Check sheet for the drawn part. Datum: minimum x, y, z corner. Units: mm. A direction names the side the tool comes from. Give positions to 0.01 mm unless a question says otherwise; leave off trailing zeros. Order: outer loops, then holes, each group sorted by start corner. A loop starts at its lowest first (then second) coordinate and runs counter-clockwise, first axis right, second up. Notation, with made-up numbers: (-7.75, -3.75) - (4.25, -3.75) arc R20 ccw to (4.25, 4.25) - close; hole circle Ø5 at (69.5, 69). An arc over 180 degrees is marked (long way). Answer as a JSON object with one key per item and string values. Group by question number.
(1) Thickness scan on line 1 (Y direction, x = 39, z = 83); line 2 (X direction, y = 2, z = 25); line 3 (X direction, y = 1, z = 66). Record the ranges inside material, lowest first.
(2) Mould release check, pull along Z, two halves, no side actions. Record for the marked faces 1, 2 and 3: +Z half, -Z half, draft (parallel to the pull), parting line (faces both ways), or undercut.
(3) Section check D-D (z = 56). Record the boundary of the cut face in (x, y).
(4) Depth check by flat-ended pin: pin 1 Ø3 at (y, z) = (21, 52) entering from -X; pin 2 Ø5 at (y, z) = (43, 66.5) entering from +X; pin 3 Ø8 at (x, y) = (78, 46) entering from -Z. Enter the tip coordinate at first touch or a pass-through.
(5) Access from +Z, -Z, +X, -X, +Y, -Y to the whole of each face (thin tool, end or side, straight path). Record for the marked faces 4 and 5.
(6) Section check C-C (x = 57). Record the boundary of the cut face in (y, z).
(7) Section check A-A (x = 25.5). Count the separate pieces of the cut face and the enclosed holes in it.
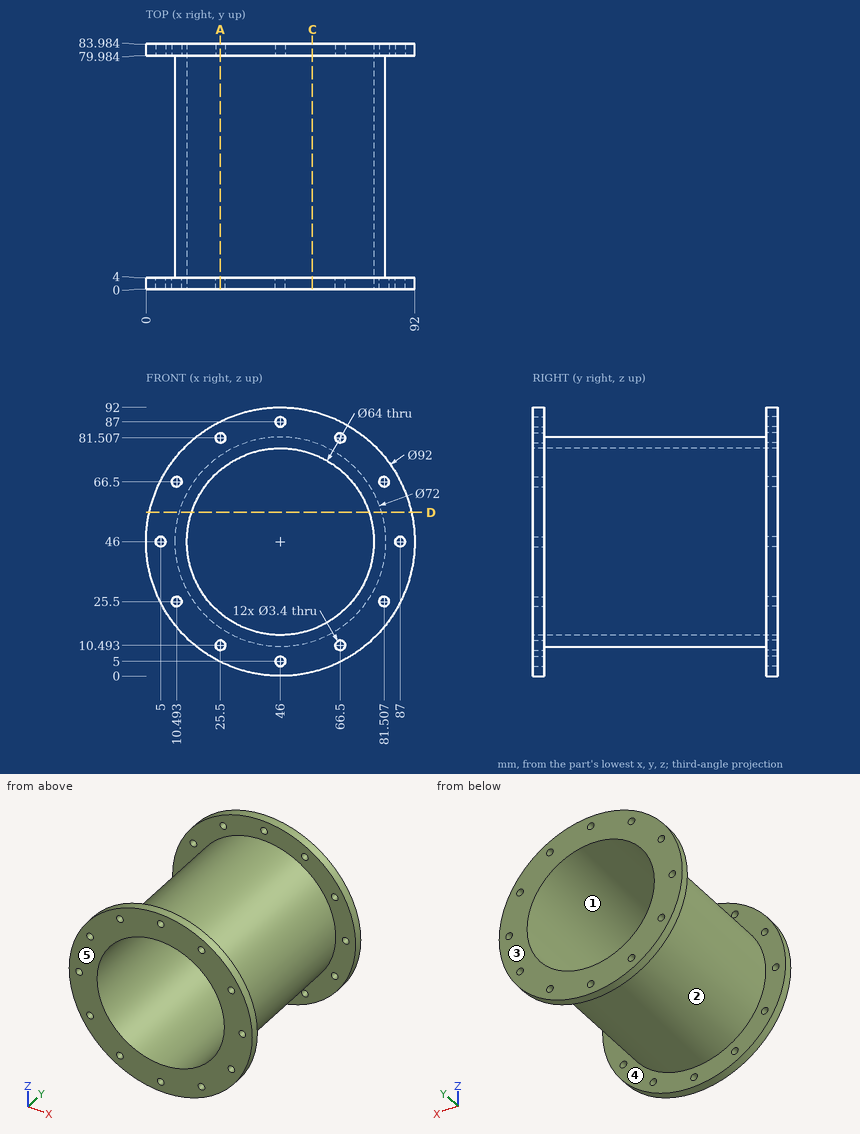
Solutions:
{
 "1": {"line 1": "y = 0 to 4, 79.98 to 83.98", "line 2": "x = 5.07 to 8.87, 12.12 to 21.85, 70.15 to 79.88, 83.13 to 86.93", "line 3": "x = 4.58 to 8.87, 12.12 to 21.02, 70.98 to 79.88, 83.13 to 87.42"},
 "2": {"face 1": "undercut", "face 2": "parting line", "face 3": "draft"},
 "3": {"outline": "(1.1, 0) - (15.6, 0) - (15.6, 83.98) - (1.1, 83.98) - (1.1, 79.98) - (11.42, 79.98) - (11.42, 4) - (1.1, 4) - close; (76.4, 0) - (90.9, 0) - (90.9, 4) - (80.58, 4) - (80.58, 79.98) - (90.9, 79.98) - (90.9, 83.98) - (76.4, 83.98) - close"},
 "4": {"pin 1": "stops at x = 10.28", "pin 2": "stops at x = 77.18", "pin 3": "stops at z = 23.37"},
 "5": {"face 4": "none", "face 5": "+Z, -Z, +X, -X, -Y"},
 "6": {"outline": "(0, 1.33) - (4, 1.33) - (4, 11.72) - (79.98, 11.72) - (79.98, 1.33) - (83.98, 1.33) - (83.98, 15.95) - (0, 15.95) - close; (0, 76.05) - (83.98, 76.05) - (83.98, 90.67) - (79.98, 90.67) - (79.98, 80.28) - (4, 80.28) - (4, 90.67) - (0, 90.67) - close"},
 "7": {"separate pieces": "6", "enclosed holes": "0"}
}
